Part model, mm, in its own coordinate system. A direction names the side the tool comes from. Round coordinates to 2 decimals unless told otherwise and drop trailing zeros. Write each loop counter-clockwise with the first axis right and the second up, starting at its lowest first coordinate (ties: lowest second). Pieces come first, ordered by that corner, then holes.
```python
from build123d import *

# Parameters (mm, degrees)
SKETCH1_W           = 25.4
SKETCH1_H           = 748.388181024
BOSS_EXTRUDE1_DEPTH = 25.4
SKETCH2_W           = 19.05
SKETCH2_H           = 19.05
CUT_EXTRUDE1_DEPTH  = 750.249751082


with BuildPart() as part:
    # Sketch1 → Boss-Extrude1 (new body)
    with BuildSketch(Plane(origin=(0, 0, 0), x_dir=(1, 0, 0), z_dir=(0, 1, 0))):
        with Locations((-12.7, 0)):
            Rectangle(SKETCH1_W, SKETCH1_H)
    extrude(amount=BOSS_EXTRUDE1_DEPTH)

    # Sketch2 → Cut-Extrude1 (cut, through all)
    with BuildSketch(Plane.XY.offset(374.194090512)):
        with Locations((-12.7, 12.7)):
            Rectangle(SKETCH2_W, SKETCH2_H)
    extrude(amount=-CUT_EXTRUDE1_DEPTH, mode=Mode.SUBTRACT)


solid = part.part
```
Q1. Mould opens along X. For faces 1 (the flat face through (-25.4, 13, 5)), 2 (the flat face through (-3.175, 13, 5)), 3 (the flat face through (-2, 13, 374.194)) say: +X half, -X half, draft (parallel to the pull), parting line (faces both ways), or undercut.
Values follow:
face 1: -X half
face 2: undercut
face 3: draft
Q2. Cut at C-C on y = 8. Write the cut outline in (x, z) (3 decimals).
Values follow:
outline: (-25.4, -374.194) - (-22.225, -374.194) - (-22.225, 374.194) - (-25.4, 374.194) - close; (-3.175, -374.194) - (0, -374.194) - (0, 374.194) - (-3.175, 374.194) - close
Q3. Cut at B-B on x = -7.5. Write the cut outline in (y, z) (3 decimals).
Values follow:
outline: (0, -374.194) - (3.175, -374.194) - (3.175, 374.194) - (0, 374.194) - close; (22.225, -374.194) - (25.4, -374.194) - (25.4, 374.194) - (22.225, 374.194) - close
Q4. Which spindle directions (+Z, -Z, +X, -X, +Y, -Y) get a long thin tool onto all of the face, cutting with end or side? Do faces 4 (the flat face through (-2, 13, -374.194)), 5 (the flat face through (-13, 22.225, 5)). Say none if no direction does.
Values follow:
face 4: -Z, +X, -X, +Y, -Y
face 5: +Z, -Z
Q5. Cut at A-A on z = -141. Write the cut outline in (x, y) (3 decimals), plus the area to 3 significant figures.
Values follow:
outline: (-25.4, 0) - (0, 0) - (0, 25.4) - (-25.4, 25.4) - close; hole (-22.225, 3.175) - (-3.175, 3.175) - (-3.175, 22.225) - (-22.225, 22.225) - close
area: 282 mm2
Q6. Wall check: L1, parallel to X at y = 14, z = 231.5 (3 decimals); L2, parallel to Y at x = -20, z = -215.5 (3 decimals). Give the ranges that are in metal, low to high.
Values follow:
L1: x = -25.4 to -22.225, -3.175 to 0
L2: y = 0 to 3.175, 22.225 to 25.4
Q7. Drop a flat-ended pin along its axis: pin 1 (15 mm diameter, centred on y = 15.5, z = 43.5, fed in from +X). Give the stop position or say it passes through.
Values follow:
pin 1: stops at x = 0
